Geometry check sheet. Reference: the model listing, model coordinates, mm. A direction names the side the tool comes from. Give positions to 0.01 mm unless a question says otherwise; leave off trailing zeros. Order: outer loops, then holes, each group sorted by start corner. A loop starts at its lowest first (then second) coordinate and runs counter-clockwise, first axis right, second up. Notation, with made-up numbers: M 14.25,-26 L 57.25,-26 A12 ccw 57.25,-14 Z; hole C -12.5,87.5 d7. An arc over 180 degrees is marked long. Answer as a JSON object with one key per item and string values. Group by question number.
from build123d import *

# Parameters (mm, degrees)
EXTRUDE_1_DEPTH          = 32.5
SKETCH_2_R               = 1.75
CUT_EXTRUDE_1_DEPTH      = 122.727153914
SKETCH_3_R               = 26.675
CUT_EXTRUDE_2_DEPTH      = 6
CUT_EXTRUDE_3_REACH      = 133.037
SKETCH_4_R               = 1.5
SKETCH_4_R_2             = 21
SKETCH_5_R               = 4.175
CUT_EXTRUDE_4_DEPTH      = 5.2
CHAMFER_1_SIZE           = 10
CUT_EXTRUDE_START        = -9
CUT_EXTRUDE_5_DEPTH      = 9
SKETCH_7_R               = 3.25
CUT_EXTRUDE_6_DEPTH      = 3
CHAMFER_2_SIZE           = 2
PATTERN_CIRCULAR_1_COUNT = 2
PATTERN_CIRCULAR_1_ANGLE = 24
SKETCH_10_W              = 2
SKETCH_10_H              = 3
CUT_EXTRUDE_7_DEPTH      = 3
SKETCH_11_W              = 3.5
SKETCH_11_H              = 17.5
EXTRUDE_2_DEPTH          = 15
CHAMFER_3_SIZE           = 1.5
SKETCH_12_R              = 1.1
CUT_EXTRUDE_8_DEPTH      = 3
SKETCH_13_R              = 2.05
CUT_EXTRUDE_9_DEPTH      = 6.5
SKETCH_14_W              = 2
SKETCH_14_H              = 3
CUT_EXTRUDE_10_DEPTH     = 3


with BuildPart() as part:
    # Эскиз1 → Бобышка-Вытянуть1 (new, symmetric)
    with BuildSketch(Plane.XY):
        Polygon((0, 40), (0, -51), (11, -62), (73.5, -62), (73.5, -77), (4.786796564, -77), (-15, -57.213203436), (-15, 40), align=None)
    extrude(amount=EXTRUDE_1_DEPTH, both=True)

    # Эскиз2 → Вырез-Вытянуть1 (cut, through all)
    with BuildSketch(Plane.ZY.offset(15)):
        with BuildLine():
            Line((32.5, 0), (32.5, 40))
            Line((32.5, 40), (-32.5, 40))
            Line((-32.5, 40), (-32.5, 0))
            ThreePointArc((-32.5, 0), (0, 32.5), (32.5, 0))
        make_face()
        with Locations(Location((0, -13.5, 0), (0, 0, 270))):
            Circle(SKETCH_2_R)
        with Locations(Location((11.691342951, 6.75, 0), (0, 0, 270))):
            Circle(SKETCH_2_R)
        with Locations(Location((-11.691342951, 6.75, 0), (0, 0, 270))):
            Circle(SKETCH_2_R)
    extrude(amount=-CUT_EXTRUDE_1_DEPTH, mode=Mode.SUBTRACT)

    # Эскиз3 → Вырез-Вытянуть2 (cut)
    with BuildSketch(Plane.XZ.offset(77)):
        with Locations((41, 0)):
            Circle(SKETCH_3_R)
    extrude(amount=-CUT_EXTRUDE_2_DEPTH, mode=Mode.SUBTRACT)

    # Эскиз4 → Вырез-Вытянуть3 (cut, up to next)
    with BuildSketch(Plane.XZ.offset(71), mode=Mode.PRIVATE) as cut_extrude_3_sk1:
        with Locations((64.75, 0)):
            Circle(SKETCH_4_R)
    cut_extrude_3_tool1 = extrude(cut_extrude_3_sk1.sketch, amount=-CUT_EXTRUDE_3_REACH, mode=Mode.PRIVATE) & part.part
    # Эскиз4 → Вырез-Вытянуть3 (cut, up to next)
    with BuildSketch(Plane.XZ.offset(71), mode=Mode.PRIVATE) as cut_extrude_3_sk2:
        with Locations((52.875, -20.56810334)):
            Circle(SKETCH_4_R)
    cut_extrude_3_tool2 = extrude(cut_extrude_3_sk2.sketch, amount=-CUT_EXTRUDE_3_REACH, mode=Mode.PRIVATE) & part.part
    # Эскиз4 → Вырез-Вытянуть3 (cut, up to next)
    with BuildSketch(Plane.XZ.offset(71), mode=Mode.PRIVATE) as cut_extrude_3_sk3:
        with Locations((29.125, -20.56810334)):
            Circle(SKETCH_4_R)
    cut_extrude_3_tool3 = extrude(cut_extrude_3_sk3.sketch, amount=-CUT_EXTRUDE_3_REACH, mode=Mode.PRIVATE) & part.part
    # Эскиз4 → Вырез-Вытянуть3 (cut, up to next)
    with BuildSketch(Plane.XZ.offset(71), mode=Mode.PRIVATE) as cut_extrude_3_sk4:
        with Locations((17.25, 0)):
            Circle(SKETCH_4_R)
    cut_extrude_3_tool4 = extrude(cut_extrude_3_sk4.sketch, amount=-CUT_EXTRUDE_3_REACH, mode=Mode.PRIVATE) & part.part
    # Эскиз4 → Вырез-Вытянуть3 (cut, up to next)
    with BuildSketch(Plane.XZ.offset(71), mode=Mode.PRIVATE) as cut_extrude_3_sk5:
        with Locations((29.125, 20.56810334)):
            Circle(SKETCH_4_R)
    cut_extrude_3_tool5 = extrude(cut_extrude_3_sk5.sketch, amount=-CUT_EXTRUDE_3_REACH, mode=Mode.PRIVATE) & part.part
    # Эскиз4 → Вырез-Вытянуть3 (cut, up to next)
    with BuildSketch(Plane.XZ.offset(71), mode=Mode.PRIVATE) as cut_extrude_3_sk6:
        with Locations((52.875, 20.56810334)):
            Circle(SKETCH_4_R)
    cut_extrude_3_tool6 = extrude(cut_extrude_3_sk6.sketch, amount=-CUT_EXTRUDE_3_REACH, mode=Mode.PRIVATE) & part.part
    # Эскиз4 → Вырез-Вытянуть3 (cut, up to next)
    with BuildSketch(Plane.XZ.offset(71), mode=Mode.PRIVATE) as cut_extrude_3_sk7:
        with Locations((41, 0)):
            Circle(SKETCH_4_R_2)
    cut_extrude_3_tool7 = extrude(cut_extrude_3_sk7.sketch, amount=-CUT_EXTRUDE_3_REACH, mode=Mode.PRIVATE) & part.part
    add(cut_extrude_3_tool1.solids().sort_by_distance((64.75, -71, 0))[0], mode=Mode.SUBTRACT)
    add(cut_extrude_3_tool2.solids().sort_by_distance((52.875, -71, -20.568103))[0], mode=Mode.SUBTRACT)
    add(cut_extrude_3_tool3.solids().sort_by_distance((29.125, -71, -20.568103))[0], mode=Mode.SUBTRACT)
    add(cut_extrude_3_tool4.solids().sort_by_distance((17.25, -71, 0))[0], mode=Mode.SUBTRACT)
    add(cut_extrude_3_tool5.solids().sort_by_distance((29.125, -71, 20.568103))[0], mode=Mode.SUBTRACT)
    add(cut_extrude_3_tool6.solids().sort_by_distance((52.875, -71, 20.568103))[0], mode=Mode.SUBTRACT)
    add(cut_extrude_3_tool7.solids().sort_by_distance((41, -71, 0))[0], mode=Mode.SUBTRACT)

    # Эскиз5 → Вырез-Вытянуть4 (cut)
    with BuildSketch(Plane(origin=(0, 0, 0), x_dir=(0, 0, -1), z_dir=(1, 0, 0))):
        with Locations(Location((0, 0, 0), (0, 0, 90))):
            Circle(SKETCH_5_R)
    extrude(amount=-CUT_EXTRUDE_4_DEPTH, mode=Mode.SUBTRACT)

    # Фаска1
    chamfer_1_edges = [part.edges().sort_by_distance(p)[0] for p in [
        (73.5, -69.5, 32.5),
        (73.5, -69.5, -32.5),
    ]]
    chamfer(chamfer_1_edges, length=CHAMFER_1_SIZE)

    # Эскиз6 → Вырез-Вытянуть5 (cut)
    with BuildSketch(Plane.XZ.offset(71).offset(CUT_EXTRUDE_START)):
        with BuildLine():
            ThreePointArc((34, 19.798989873), (41, 21), (48, 19.798989873))
            Line((48, 19.798989873), (48, 25.740155885))
            ThreePointArc((48, 25.740155885), (41, 26.675), (34, 25.740155885))
            Line((34, 25.740155885), (34, 19.798989873))
        make_face()
    extrude(amount=CUT_EXTRUDE_5_DEPTH, mode=Mode.SUBTRACT)

    # Эскиз7 → Вырез-Вытянуть6 (cut)
    with BuildSketch(Plane.ZY.offset(15)):
        with Locations(Location((11.691342951, 6.75, 0), (0, 0, 270))):
            Circle(SKETCH_7_R)
        with Locations(Location((0, -13.5, 0), (0, 0, 270))):
            Circle(SKETCH_7_R)
        with Locations(Location((-11.691342951, 6.75, 0), (0, 0, 270))):
            Circle(SKETCH_7_R)
    extrude(amount=-CUT_EXTRUDE_6_DEPTH, mode=Mode.SUBTRACT)

    # Фаска2
    chamfer_2_edges = [part.edges().sort_by_distance(p)[0] for p in [
        (73.5, -77, 0),
        (34.143398282, -77, -32.5),
        (68.5, -77, 27.5),
        (68.5, -77, -27.5),
        (-5.106601718, -67.106601718, -32.5),
        (-5.106601718, -67.106601718, 32.5),
        (34.143398282, -77, 32.5),
        (-15, -28.606601718, -32.5),
        (-15, -28.606601718, 32.5),
        (-15, 32.5, 0),
    ]]
    chamfer(chamfer_2_edges, length=CHAMFER_2_SIZE)

    # Эскиз9 → Вырез-Повернуть1 (revolve, cut)
    with BuildSketch(Plane(origin=(-6.5, 0, 0), x_dir=(0, 0, -1), z_dir=(1, 0, 0))):
        Polygon((-19.70026884, 15.391536883), (-18.438162816, 17.006958928), (-24.742248845, 21.932250731), (-26.004354869, 20.316828686), align=None)
    cut_revolve_1 = revolve(axis=Axis((-6.5, 0, 0), (0, 0.6156614753256564, 0.7880107536067235)), mode=Mode.SUBTRACT)

    # Круговой массив1: Вырез-Повернуть1 ×2 about axis
    pattern_circular_1_axis = Axis((73.5, 0, 0), (1, 0, 0))
    for i in range(1, PATTERN_CIRCULAR_1_COUNT):
        add(cut_revolve_1.rotate(pattern_circular_1_axis, i * PATTERN_CIRCULAR_1_ANGLE / (PATTERN_CIRCULAR_1_COUNT - 1)), mode=Mode.SUBTRACT)

    # Эскиз10 → Вырез-Вытянуть7 (cut)
    with BuildSketch(Plane(origin=(0, 0, 0), x_dir=(0, 0, -1), z_dir=(1, 0, 0))):
        with Locations((0, 31.5)):
            Rectangle(SKETCH_10_W, SKETCH_10_H)
    extrude(amount=-CUT_EXTRUDE_7_DEPTH, mode=Mode.SUBTRACT)

    # Эскиз11 → Бобышка-Вытянуть2 (add)
    with BuildSketch(Plane.XZ.offset(77)):
        with Locations((73.25, 0)):
            Rectangle(SKETCH_11_W, SKETCH_11_H)
    extrude(amount=-EXTRUDE_2_DEPTH)

    # Фаска3
    chamfer_3_edges = [part.edges().sort_by_distance(p)[0] for p in [
        (72.5, -76, -8.75),
        (73.5, -68.5, -8.75),
        (72.5, -76, 8.75),
        (73.5, -68.5, 8.75),
    ]]
    chamfer(chamfer_3_edges, length=CHAMFER_3_SIZE - 0.0001)  # a hair under: the kernel refuses the full size

    # Эскиз12 → Вырез-Вытянуть8 (cut)
    with BuildSketch(Plane(origin=(75, 0, 0), x_dir=(0, 0, -1), z_dir=(1, 0, 0))):
        with Locations(Location((0, -72.5, 0), (0, 0, 90))):
            Circle(SKETCH_12_R)
    extrude(amount=-CUT_EXTRUDE_8_DEPTH, mode=Mode.SUBTRACT)

    # Эскиз13 → Вырез-Вытянуть9 (cut)
    with BuildSketch(Plane(origin=(75, 0, 0), x_dir=(0, 0, -1), z_dir=(1, 0, 0))):
        with Locations(Location((6, -72.5, 0), (0, 0, 90))):
            Circle(SKETCH_13_R)
    extrude(amount=-CUT_EXTRUDE_9_DEPTH, mode=Mode.SUBTRACT)

    # Эскиз14 → Вырез-Вытянуть10 (cut)
    with BuildSketch(Plane.XZ.offset(77)):
        with Locations((41, 31)):
            Rectangle(SKETCH_14_W, SKETCH_14_H)
    extrude(amount=-CUT_EXTRUDE_10_DEPTH, mode=Mode.SUBTRACT)


solid = part.part
1. Access from +Z, -Z, +X, -X, +Y, -Y to the whole of each face (thin tool, end or side, straight path). Record for faces 1 (the flat face through (73.5, -68, 16)), 2 (the flat face through (48, -66, 23)), 3 (the flat face through (57, -62, -14)), 4 (the flat face through (-5.2, 0, 0)), 5 (the flat face through (-6.529, 15.414, 19.683)).
2. Depth check by flat-ended pin: pin 1 (1.5 mm diameter, centred on x = 74.5, y = -67, fed in from +Z); pin 2 (0.6 mm diameter, centred on x = 40.5, y = -75.5, fed in from +Z); pin 3 (3.5 mm diameter, centred on y = -69, z = -16.5, fed in from +X). Enter the tip coordinate at first touch or a pass-through.
3. Cross-section at B-B (x = 17.25). Record the cut outline in (y, z).
4. Cross-section at A-A (y = -13.5). Record the cut outline in (x, z).
5. Thickness scan on line 1 along Z through (x, y) = (41, -72.35) (3 decimals); line 2 along Z through (x, y) = (-6.75, 6.75); line 3 along Y through (x, z) = (14, 2). Record the ranges inside material, lowest first. Write a range as [from, to].
6. Cross-section at C-C (y = -41). Record the cut outline in (x, z).
7. Release check for a two-part mould opening along Y. For faces 6 (the flat face through (34, -66, 23)), 7 (the cylindrical face through (-6.591, 32.492, -0.715)), 8 (the cylindrical face through (-13.52, 7.17, -8.47)) record: released by +Y, released by -Y, zero draft, split by the parting line, or undercut.
Report:
{
 "1": {"face 1": "+Z, +X, +Y, -Y", "face 2": "+Y, -Y", "face 3": "+Z, -Z, +X, +Y", "face 4": "+X", "face 5": "none"},
 "2": {"pin 1": "stops at z = 10", "pin 2": "stops at z = 29.5", "pin 3": "stops at x = 73.5"},
 "3": {"outline": "M -77,-30.5 L -75,-32.5 L -62,-32.5 L -62,-1.5 L -71,-1.5 L -71,-12.14 L -77,-12.14 Z; M -77,12.14 L -71,12.14 L -71,1.5 L -62,1.5 L -62,32.5 L -75,32.5 L -77,30.5 Z"},
 "4": {"outline": "M -15,-30.5 L -13,-32.5 L 0,-32.5 L 0,-1.75 L -12,-1.75 L -12,-3.25 L -15,-3.25 Z; M -15,3.25 L -12,3.25 L -12,1.75 L 0,1.75 L 0,32.5 L -13,32.5 L -15,30.5 Z"},
 "5": {"line 1": "z = [-32.5, -26.675], [26.675, 32.5]", "line 2": "z = [-31.79, -13.44], [-9.94, 9.94], [13.44, 24.08]", "line 3": "y = [-77, -62]"},
 "6": {"outline": "M -15,-30.5 L -13,-32.5 L 0,-32.5 L 0,32.5 L -13,32.5 L -15,30.5 Z"},
 "7": {"face 6": "zero draft", "face 7": "released by +Y", "face 8": "undercut"}
}
